from build123d import *


with BuildPart() as part:
    # Szkic1 → Obrót1 (revolve)
    with BuildSketch(Plane(origin=(0, 0, 0), x_dir=(0, 0, -1), z_dir=(1, 0, 0)), mode=Mode.PRIVATE) as obr_t1_sk:
        Polygon((-31.2, -2.5), (-31.2, -2.4), (-30.5, -2.4), (-30.5, -2.5), (30.5, -2.5), (30.5, -2.4), (31.2, -2.4), (31.2, -2.5), (32.5, -2.5), (32.5, 0), (-32.5, 0), (-32.5, -2.5), align=None)
    revolve(obr_t1_sk.sketch.rotate(Axis((0, 0, 32.5), (0, 0, -1)), 270), axis=Axis((0, 0, 32.5), (0, 0, -1)))


solid = part.part
Verification items for the finished model (mm, model axes). Coordinates: 2 decimals unless noted, no trailing zeros. Order: outer loops, then holes, each group sorted by start corner. A loop starts at its lowest first (then second) coordinate and runs counter-clockwise, first axis right, second up.
Item 1: Section check B-B, the plane y = -1.7. Enter the section's corners in (x, z).
Filled in:
outline: (-1.83, -32.5) - (1.83, -32.5) - (1.83, -31.2) - (1.69, -31.2) - (1.69, -30.5) - (1.83, -30.5) - (1.83, 30.5) - (1.69, 30.5) - (1.69, 31.2) - (1.83, 31.2) - (1.83, 32.5) - (-1.83, 32.5) - (-1.83, 31.2) - (-1.69, 31.2) - (-1.69, 30.5) - (-1.83, 30.5) - (-1.83, -30.5) - (-1.69, -30.5) - (-1.69, -31.2) - (-1.83, -31.2) - close
Item 2: Section check C-C, the plane z = -10. Enter the section's corners in (x, y), then the cut area to 3 significant figures.
Filled in:
outline: circle Ø5 at (0, 0)
area: 19.6 mm2
Item 3: Release check for a two-part mould opening along Z. For faces 1 (the face through (0, 0, 32.5)), 2 (the face through (1.29, -2.024, -30.855)), 3 (the face through (0, 0, -32.5)), 4 (the face through (1.29, -2.024, 30.845)) record: +Z half, -Z half, draft (parallel to the pull), parting line (faces both ways), or undercut.
Filled in:
face 1: +Z half
face 2: undercut
face 3: -Z half
face 4: undercut
Item 4: Section check A-A, the plane x = 1.45. Enter the section's corners in (y, z), then the cut area to 3 significant figures.
Filled in:
outline: (-2.04, -32.5) - (2.04, -32.5) - (2.04, -31.2) - (1.91, -31.2) - (1.91, -30.5) - (2.04, -30.5) - (2.04, 30.5) - (1.91, 30.5) - (1.91, 31.2) - (2.04, 31.2) - (2.04, 32.5) - (-2.04, 32.5) - (-2.04, 31.2) - (-1.91, 31.2) - (-1.91, 30.5) - (-2.04, 30.5) - (-2.04, -30.5) - (-1.91, -30.5) - (-1.91, -31.2) - (-2.04, -31.2) - close
area: 264 mm2
Item 5: Depth check by flat-ended pin: pin 1 (1.5 mm diameter, centred on x = -1.5, z = 4.5, fed in from -Y); pin 2 (2 mm diameter, centred on x = 2, z = 2, fed in from -Y). Enter the tip coordinate at first touch or a pass-through.
Filled in:
pin 1: stops at y = -2.38
pin 2: stops at y = -2.29
Item 6: Material ranges on L1, parallel to X at y = -0.7, z = -2; L2, parallel to X at y = 1.7, z = -22; L3, parallel to Y at x = 1.35, z = 21, recorded low to high.
Filled in:
L1: x = -2.4 to 2.4
L2: x = -1.83 to 1.83
L3: y = -2.1 to 2.1
